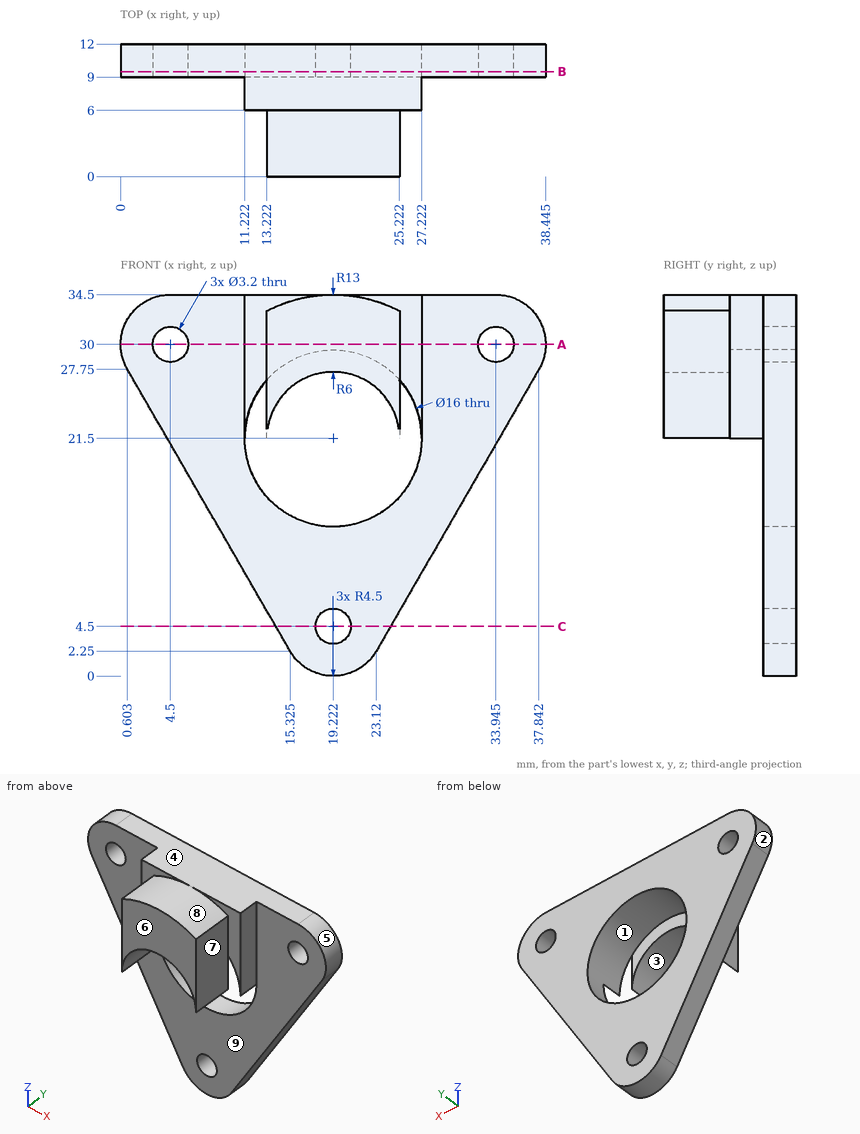
The figure shows three views and two pictorial views of one solid part (mm, origin at its lowest corner). Answer the questions. A direction names the side the tool comes from. Give positions to 0.01 mm unless a question says otherwise; leave off trailing zeros. Order: outer loops, then holes, each group sorted by start corner. A loop starts at its lowest first (then second) coordinate and runs counter-clockwise, first axis right, second up. Notation, with made-up numbers: M -29.75,-7.5 L 27.25,-7.5 A29 cw 27.25,27.5 Z; hole C 36,-37 d10. An arc over 180 degrees is marked long. Return JSON: item names as keys, results as strings.
1) Straight lines are drawn through the part: line 1 along X through (y, z) = (10.2, 30) (1 decimal); line 2 along Y through (x, z) = (27.5, 15); line 3 along Y through (x, z) = (13, 29). For each, find the intervals that lie inside material, in ascending order. Write a range as [from, to].
Resolved:
{"line 1": "[0, 2.9], [6.1, 32.3], [35.5, 38.4]", "line 2": "[9, 12]", "line 3": "[6, 12]"}
2) Each of these flat-tipped pins is pushed along its axis until it touches: pin 1 (1.5 mm diameter, centred on x = 12, y = 3, fed in from +Z); pin 2 (13 mm diameter, centred on x = 19.22, z = 21.5, fed in from +Y); pin 3 (1.8 mm diameter, centred on y = 2.5, z = 26, fed in from +X); pin 4 (1.8 mm diameter, centred on y = 3, z = 26.5, fed in from -X). Where does it stop, or does it pass through?
Resolved:
{"pin 1": "through", "pin 2": "y = 6", "pin 3": "x = 25.22", "pin 4": "x = 13.22"}
3) For a pull along X with two mould halves and no side action, classify the marked faces 1, 2, 3 and 4 as +X half, -X half, draft (parallel to the pull), parting line (faces both ways), or undercut.
Resolved:
{"face 1": "undercut", "face 2": "-X half", "face 3": "undercut", "face 4": "draft"}
4) A tool of negligible diameter and unlimited length cuts with its end or side. For the marked faces 5, 6, 7, 8 and 9, from which of +Z, -Z, +X, -X, +Y, -Y can it reach the whole face along a straight path? Write none if from no direction.
Resolved:
{"face 5": "+X, +Y, -Y", "face 6": "+Z, -Z, +X, -X, -Y", "face 7": "+Z, -Z, +X, -Y", "face 8": "+Z, -Y", "face 9": "-Z, -Y"}
5) Section C-C, the plane z = 4.5 is taken. Write down the section's boundary in (x, y), plus the area to 3 significant figures.
Resolved:
{"outline": "M 14.03,9 L 17.62,9 L 17.62,12 L 14.03,12 Z; M 20.82,9 L 24.42,9 L 24.42,12 L 20.82,12 Z", "area": "21.6 mm^2"}
6) Section A-A, the plane z = 30 is taken. Write down the section's boundary in (x, y) (1 decimal).
Resolved:
{"outline": "M 0,9 L 2.9,9 L 2.9,12 L 0,12 Z; M 6.1,9 L 11.2,9 L 11.2,6 L 13.2,6 L 13.2,0 L 25.2,0 L 25.2,6 L 27.2,6 L 27.2,9 L 32.3,9 L 32.3,12 L 6.1,12 Z; M 35.5,9 L 38.4,9 L 38.4,12 L 35.5,12 Z"}
7) Section B-B, the plane y = 9.5 is taken. Give the number of separate pieces and of enclosed holes in the cut face.
Resolved:
{"separate pieces": "1", "enclosed holes": "4"}
